Source: three-view drawing plus pictorial views. Frame: mm from the lowest corner of the part. A direction names the side the tool comes from. Give positions to 0.01 mm unless a question says otherwise; leave off trailing zeros. Order: outer loops, then holes, each group sorted by start corner. A loop starts at its lowest first (then second) coordinate and runs counter-clockwise, first axis right, second up.
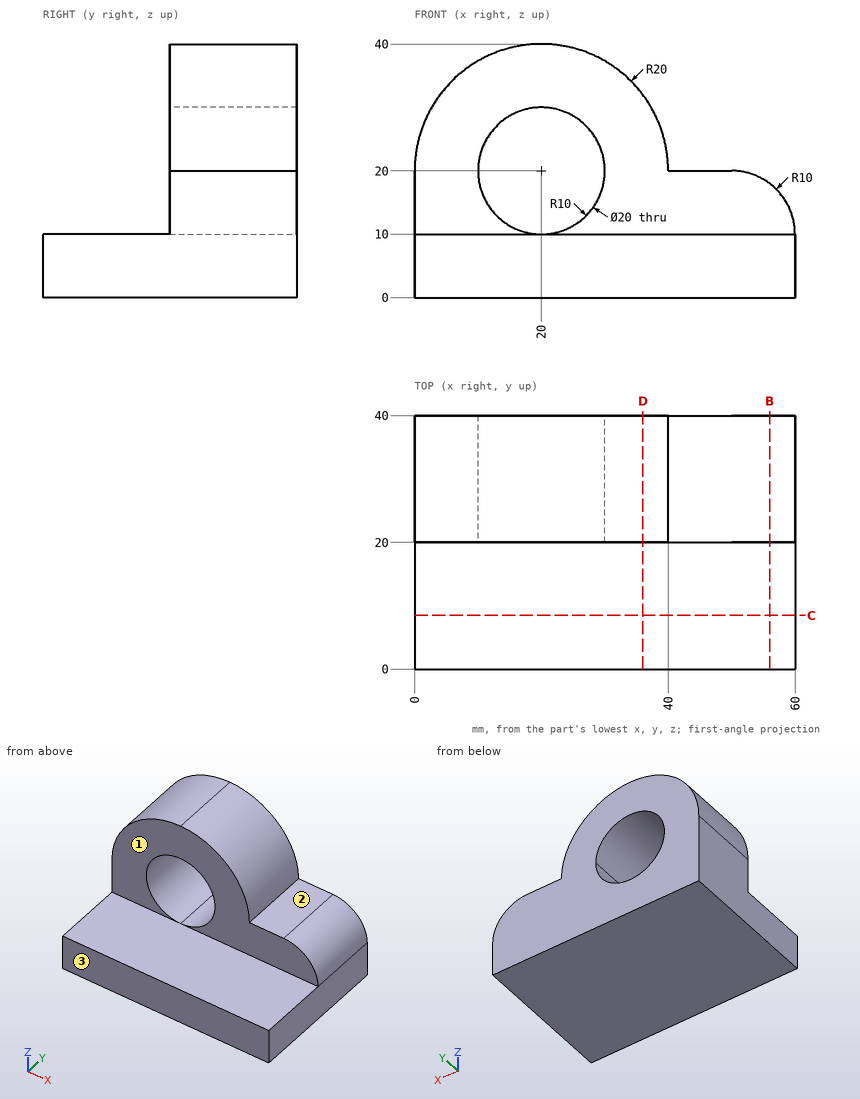
1) First-contact query: pin 1 Ø16 at (x, y) = (37, 5.5) entering from +Z; pin 2 Ø3 at (x, y) = (45, 25.5) entering from +Z; pin 3 Ø5 at (y, z) = (18.5, 25.5) entering from +X; pin 4 Ø2 at (x, y) = (21, 9.5) entering from -Z. Flat tips, straight axial feed; report the tip coordinate or a pass-through.
Checks:
pin 1: stops at z = 10
pin 2: stops at z = 20
pin 3: stops at x = 39.69
pin 4: stops at z = 0
2) Section query D-D on x = 36. Output: boundary loops of the cut face in (y, z).
Checks:
outline: (0, 0) - (40, 0) - (40, 32) - (20, 32) - (20, 10) - (0, 10) - close
3) Ray query, L1, parallel to Z at x = 20, y = 28; L2, parallel to Z at x = 34.5, y = 15; L3, parallel to Y at x = 10.5, z = 12.5. Return the intervals inside material, ascending.
Checks:
L1: z = 0 to 10, 30 to 40
L2: z = 0 to 10
L3: y = 20 to 40
4) Reachability of the marked faces 1, 2 and 3 from +Z, -Z, +X, -X, +Y, -Y: full face, straight path, thin tool, end or side. Return the list, or none.
Checks:
face 1: +Z, +X, -X, -Y
face 2: +Z, +X, +Y, -Y
face 3: +Z, -Z, +X, -X, -Y
5) Section query C-C on y = 8.5. Output: boundary loops of the cut face in (x, z).
Checks:
outline: (0, 0) - (60, 0) - (60, 10) - (0, 10) - close
6) Section query B-B on x = 56. Output: boundary loops of the cut face in (y, z).
Checks:
outline: (0, 0) - (40, 0) - (40, 18) - (20, 18) - (20, 10) - (0, 10) - close
